Geometry check sheet. Reference: the model listing, model coordinates, mm. A direction names the side the tool comes from. Round coordinates to 2 decimals unless told otherwise and drop trailing zeros. Write each loop counter-clockwise with the first axis right and the second up, starting at its lowest first coordinate (ties: lowest second). Pieces come first, ordered by that corner, then holes. Notation, with made-up numbers: M 88,-19.75 L 121,-19.75 A17 cw 121,-4.75 Z; hole C -3.5,-15 d1. An arc over 180 degrees is marked long. Use a Markdown table: item, result.
```python
from build123d import *

# Parameters (mm, degrees)
F0_R     = 3.175
F1_DEPTH = 76.2
F3_DEPTH = 25.4
F5_DEPTH = 50.8


with BuildPart() as f1:
    # F0 (on Top) → F1 (new body)
    with BuildSketch(Plane.XY):
        with Locations((-45.71999982, 18.5057148337)):
            Circle(F0_R)
    extrude(amount=F1_DEPTH)

    # F2 (on face) → F3 (join)
    with BuildSketch(Plane.XY.offset(76.2)):
        with BuildLine():
            Line((-43.17999982, 20.4107148337), (-48.25999982, 20.4107148337))
            ThreePointArc((-48.25999982, 20.4107148337), (-46.7240229771, 15.4936453624), (-42.54499982, 18.5057148337))
            ThreePointArc((-42.54499982, 18.5057148337), (-42.7079303487, 19.5097379908), (-43.17999982, 20.4107148337))
        make_face()
    extrude(amount=F3_DEPTH)

    # F4 (on face) → F5 (cut)
    with BuildSketch(Plane(origin=(0, 0, 0), x_dir=(1, 0, 0), z_dir=(0, 0, -1))):
        with BuildLine():
            Line((-47.30749982, -15.7560841767), (-47.30749982, -21.2553454908))
            ThreePointArc((-47.30749982, -21.2553454908), (-45.71999982, -21.6807148337), (-44.13249982, -21.2553454908))
            Line((-44.13249982, -21.2553454908), (-44.13249982, -15.7560841767))
            ThreePointArc((-44.13249982, -15.7560841767), (-45.71999982, -15.3307148337), (-47.30749982, -15.7560841767))
        make_face()
    extrude(amount=-F5_DEPTH, mode=Mode.SUBTRACT)


solid = f1.part
```
Item 1: Access from +Z, -Z, +X, -X, +Y, -Y to the whole of each face (thin tool, end or side, straight path). Record for faces 3 (the face through (-47.307, 18, 25)), 4 (the face through (-46, 18, 101.6)), 5 (the face through (-46, 20.411, 89)).
Outcome:
| item | result |
|---|---|
| face 3 | -Z, +Y, -Y |
| face 4 | +Z, +X, -X, +Y, -Y |
| face 5 | +Z, +X, -X, +Y |
Item 2: Material ranges on line 1 along Z through (x, y) = (-44.25, 17.5); line 2 along Z through (x, y) = (-47, 20.75); line 3 along X through (y, z) = (20.75, 26), recorded low to high. Write a range as from..to.
Outcome:
| item | result |
|---|---|
| line 1 | z = 50.8..101.6 |
| line 2 | z = 50.8..76.2 |
| line 3 | x = -47.97..-47.31, -44.13..-43.47 |
Item 3: Cross-section at A-A, the plane z = 78.5. Record the cut outline in (x, y) (3 decimals).
Outcome:
| item | result |
|---|---|
| outline | M -48.26,20.411 A3.175 ccw long -43.18,20.411 Z |
Item 4: Cross-section at C-C, the plane z = 52.5. Record the cut outline in (x, y) (3 decimals), and give its area (3 significant figures).
Outcome:
| item | result |
|---|---|
| outline | C -45.72,18.506 d6.35 |
| area | 31.7 mm2 |
Item 5: Cross-section at B-B, the plane x = -45.72. Record the cut outline in (y, z), and give its area (3 significant figures).
Outcome:
| item | result |
|---|---|
| outline | M 15.33,50.8 L 21.68,50.8 L 21.68,76.2 L 20.41,76.2 L 20.41,101.6 L 15.33,101.6 Z |
| area | 290 mm2 |
Item 6: Mould release check, pull along X, two halves, no side actions. Record for faces 1 (the face through (-43.5, 18.5, 0)), 2 (the face through (-46, 18, 50.8)): +X half, -X half, draft (parallel to the pull), parting line (faces both ways), or undercut.
Outcome:
| item | result |
|---|---|
| face 1 | draft |
| face 2 | undercut |
Item 7: Go/stop test with flat-tipped pins: pin 1 (2.5 mm diameter, centred on y = 17.5, z = 27.5, fed in from +X) (3 decimals); pin 2 (3 mm diameter, centred on y = 16, z = 18, fed in from -X); pin 3 (2.5 mm diameter, centred on x = -47, z = 86.5, fed in from +Y); pin 4 (0.6 mm diameter, centred on x = -45.5, y = 21, fed in from +Z). Record where each tip stops, or that it passes through.
Outcome:
| item | result |
|---|---|
| pin 1 | stops at x = -42.545 |
| pin 2 | stops at x = -48.73 |
| pin 3 | stops at y = 20.41 |
| pin 4 | stops at z = 76.2 |
